Work out the finished part from the listing and answer in its coordinate system (mm). A direction names the side the tool comes from. Coordinates: 2 decimals unless noted, no trailing zeros. Write each loop counter-clockwise with the first axis right and the second up, starting at its lowest first coordinate (ties: lowest second). Pieces come first, ordered by that corner, then holes. Notation, with made-up numbers: (48.5, 15) - (100.5, 15) arc R32 cw to (100.5, 47) - close; hole circle Ø8 at (65.25, -8). An arc over 180 degrees is marked (long way). Use a Markdown table: item, result. Add a question column.
(1) Find the intervals of material crossed by line 1 (Y direction, x = 5, z = -2); line 2 (X direction, y = -15.5, z = -1.85); line 3 (Z direction, x = 5, y = 1.55), in increasing order. Write a range as from..to.
(2) For a pull along X with two mould halves and no side action, classify faces 4 (the face through (10, 0, 3)), 5 (the face through (5, -20, -2)), 6 (the face through (5.672, 16.554, -1.63)) as released by +X, released by -X, zero draft, split by the parting line, or undercut.
(3) The part is cut by section A-A, the plane z = 8. Give the vertices of the cut face in (x, y), then the cut area to 3 significant figures.
(4) Given pin 1 Ø4 at (x, y) = (5, 15.5) entering from +Z; pin 2 Ø3 at (x, z) = (2, 10) entering from +Y; pin 3 Ø3 at (x, z) = (4, 4) entering from -Y, each flat-ended and moving along its own axis, determine where each tip first touches the part or whether it passes through.
(5) A tool of negligible diameter and unlimited length cuts with its end or side. For faces 1 (the face through (4.84, -16.74, -1.63)), 2 (the face through (5, 6, 5)), 3 (the face through (5, -13, 0)), from which of +Z, -Z, +X, -X, +Y, -Y can it reach the whole face along a straight path? Write none if from no direction.
(6) The part is cut by section C-C, the plane y = 0.5. Give the vertices of the cut face in (x, z).
(7) The part is cut by section B-B, the plane x = 5. Give the vertices of the cut face in (y, z), then the cut area to 3 significant figures.
(8) The part is cut by section D-D, the plane y = -15.5. Give the vertices of the cut face in (x, z), then the cut area to 3 significant figures.
from build123d import *

# Parameters (mm, degrees)
BOSS_EXTRU_1_DEPTH         = 20
ESQUISSE2_W                = 10
ESQUISSE2_H                = 13
BOSS_EXTRU_2_DEPTH         = 6
D_GAGEMENT_M41_D           = 4
D_GAGEMENT_M41_CSINK_D     = 5
D_GAGEMENT_M41_CSINK_ANGLE = 90
D_GAGEMENT_M2_51_D         = 2.5


with BuildPart() as part:
    # Esquisse1 → Boss.-Extru.1 (new body)
    with BuildSketch(Plane(origin=(0, 0, 0), x_dir=(1, 0, 0), z_dir=(0, 1, 0))):
        with BuildLine():
            Line((0, 0), (10, 0))
            Line((10, 0), (10, 3))
            ThreePointArc((10, 3), (5, 3.306020101), (0, 3))
            Line((0, 3), (0, 0))
        make_face()
    boss_extru_1 = extrude(amount=BOSS_EXTRU_1_DEPTH)

    # Esquisse2 → Boss.-Extru.2 (add)
    with BuildSketch(Plane.XZ):
        with Locations((5, 6.5)):
            Rectangle(ESQUISSE2_W, ESQUISSE2_H)
    boss_extru_2 = extrude(amount=-BOSS_EXTRU_2_DEPTH)

    # Dégagement M41 (through all)
    with Locations(Plane(origin=(0, 6, 0), x_dir=(1, 0, 0), z_dir=(0, 1, 0))):
        with Locations((5, -8)):
            d_gagement_m41 = CounterSinkHole(D_GAGEMENT_M41_D / 2, D_GAGEMENT_M41_CSINK_D / 2, counter_sink_angle=D_GAGEMENT_M41_CSINK_ANGLE)

    # Dégagement M2.51 (through all)
    with Locations(Plane(origin=(5, 15.5, -3.306020101), x_dir=(-1, 0, 0), z_dir=(0, 0, -1))):
        with Locations((0, 0)):
            d_gagement_m2_51 = Hole(D_GAGEMENT_M2_51_D / 2)

    # Symétrie1: Boss.-Extru.1, Boss.-Extru.2, Dégagement M41, Dégagement M2.51 across plane
    add(boss_extru_1.mirror(Plane(origin=(5, 0, 37.693979899), x_dir=(0, 0, 1), z_dir=(0, -1, 0))))
    add(boss_extru_2.mirror(Plane(origin=(5, 0, 37.693979899), x_dir=(0, 0, 1), z_dir=(0, -1, 0))))
    add(d_gagement_m41.mirror(Plane(origin=(5, 0, 37.693979899), x_dir=(0, 0, 1), z_dir=(0, -1, 0))), mode=Mode.SUBTRACT)
    add(d_gagement_m2_51.mirror(Plane(origin=(5, 0, 37.693979899), x_dir=(0, 0, 1), z_dir=(0, -1, 0))), mode=Mode.SUBTRACT)


solid = part.part
Model answer:
| question | item | result |
|---|---|---|
| 1 | line 1 | -20..-16.75, -14.25..14.25, 16.75..20 |
| 1 | line 2 | 0..3.75, 6.25..10 |
| 1 | line 3 | -3.31..6, 10..13 |
| 2 | face 4 | released by +X |
| 2 | face 5 | zero draft |
| 2 | face 6 | undercut |
| 3 | outline | (0, -6) - (2.5, -6) - (3, -5.5) - (3, 5.5) - (2.5, 6) - (0, 6) - close; (7, -5.5) - (7.5, -6) - (10, -6) - (10, 6) - (7.5, 6) - (7, 5.5) - close |
| 3 | area | 71.5 mm^2 |
| 4 | pin 1 | z = 0 |
| 4 | pin 2 | y = 6 |
| 4 | pin 3 | y = -6 |
| 5 | face 1 | +Z, -Z |
| 5 | face 2 | +Z, +X, -X, +Y |
| 5 | face 3 | +Z, +X, -X, -Y |
| 6 | outline | (0, -3) arc R41 ccw to (10, -3) - (10, 13) - (0, 13) - close; hole circle Ø4 at (5, 8) |
| 7 | outline | (-20, -3.31) - (-16.75, -3.31) - (-16.75, 0) - (-20, 0) - close; (-14.25, -3.31) - (14.25, -3.31) - (14.25, 0) - (6, 0) - (6, 5.5) - (5.5, 6) - (-5.5, 6) - (-6, 5.5) - (-6, 0) - (-14.25, 0) - close; (-6, 10.5) - (-5.5, 10) - (5.5, 10) - (6, 10.5) - (6, 13) - (-6, 13) - close; (16.75, -3.31) - (20, -3.31) - (20, 0) - (16.75, 0) - close |
| 7 | area | 223 mm^2 |
| 8 | outline | (0, -3) arc R41 ccw to (3.75, -3.29) - (3.75, 0) - (0, 0) - close; (6.25, -3.29) arc R41 ccw to (10, -3) - (10, 0) - (6.25, 0) - close |
| 8 | area | 23.8 mm^2 |
